For this review, take the finished solid that the model builds, in its own axes (mm). A direction names the side the tool comes from. Give positions to 0.01 mm unless a question says otherwise; leave off trailing zeros. Write each loop counter-clockwise with the first axis right and the second up, starting at its lowest first coordinate (ties: lowest second). Pieces come first, ordered by that corner, then holes. Notation, with made-up numbers: M 28,39.5 L 38,39.5 A21 ccw 38,58.5 Z; hole C -33.5,62.25 d2. An arc over 180 degrees is marked long. Answer as a JSON object with one key per item and string values. Group by question number.
```python
from build123d import *

# Parameters (mm, degrees)
SKETCH_1_W          = 95
SKETCH_1_H          = 45.5
EXTRUDE_1_DEPTH     = 2
SKETCH_2_W          = 7
SKETCH_2_H          = 2
CUT_EXTRUDE_1_DEPTH = 106.352978126
SKETCH_3_R          = 0.5
CUT_EXTRUDE_2_DEPTH = 106.352978126
SKETCH_5_W          = 13.5
SKETCH_5_H          = 24.5
CUT_EXTRUDE_3_DEPTH = 106.352978126
SKETCH_6_W          = 2
SKETCH_6_H          = 7
EXTRUDE_2_DEPTH     = 2
SKETCH_7_R          = 1.6
CUT_EXTRUDE_4_DEPTH = 2


with BuildPart() as part:
    # 草图1 → 凸台-拉伸1 (new body)
    with BuildSketch(Plane.XY):
        with Locations((47.5, 22.75)):
            Rectangle(SKETCH_1_W, SKETCH_1_H)
    extrude(amount=EXTRUDE_1_DEPTH)

    # 草图2 → 切除-拉伸1 (cut, through all)
    with BuildSketch(Plane.XY.offset(2)):
        with Locations((58.5, 44.5)):
            Rectangle(SKETCH_2_W, SKETCH_2_H)
        with Locations((36.5, 44.5)):
            Rectangle(SKETCH_2_W, SKETCH_2_H)
        with Locations((14.5, 44.5)):
            Rectangle(SKETCH_2_W, SKETCH_2_H)
        with Locations((80.5, 44.5)):
            Rectangle(SKETCH_2_W, SKETCH_2_H)
        with Locations((36.5, 1)):
            Rectangle(SKETCH_2_W, SKETCH_2_H)
        with Locations((58.5, 1)):
            Rectangle(SKETCH_2_W, SKETCH_2_H)
        with Locations((80.5, 1)):
            Rectangle(SKETCH_2_W, SKETCH_2_H)
    extrude(amount=-CUT_EXTRUDE_1_DEPTH, mode=Mode.SUBTRACT)

    # 草图3 → 切除-拉伸2 (cut, through all)
    with BuildSketch(Plane.XY.offset(2)):
        with Locations((11, 43.5)):
            Circle(SKETCH_3_R)
    cut_extrude_2 = extrude(amount=-CUT_EXTRUDE_2_DEPTH, mode=Mode.SUBTRACT)

    # 草图5 → 切除-拉伸3 (cut, through all)
    with BuildSketch(Plane.XY.offset(2)):
        with Locations((6.75, 12.25)):
            Rectangle(SKETCH_5_W, SKETCH_5_H)
    extrude(amount=-CUT_EXTRUDE_3_DEPTH, mode=Mode.SUBTRACT)

    # 草图6 → 凸台-拉伸2 (add)
    with BuildSketch(Plane.XY.offset(2)):
        with Locations((-1, 35)):
            Rectangle(SKETCH_6_W, SKETCH_6_H)
        with Locations((96, 32)):
            Rectangle(SKETCH_6_W, SKETCH_6_H)
        with Locations((96, 13.5)):
            Rectangle(SKETCH_6_W, SKETCH_6_H)
    extrude(amount=-EXTRUDE_2_DEPTH)

    # 草图阵列1: 切除-拉伸2 at 19 more places
    with Locations((7, 0, 0), (22, 0, 0), (29, 0, 0), (44, 0, 0), (51, 0, 0), (66, 0, 0), (73, 0, 0), (73, -41.5, 0), (66, -41.5, 0), (51, -41.5, 0), (44, -41.5, 0), (29, -41.5, 0), (22, -41.5, 0), (-11, -12, 0), (84, -8, 0), (-11, -5, 0), (84, -15, 0), (84, -26.5, 0), (84, -33.5, 0)):
        add(cut_extrude_2, mode=Mode.SUBTRACT)

    # 草图7 → 切除-拉伸4 (cut)
    with BuildSketch(Plane.XY.offset(2)):
        with Locations((6.75, 40.5)):
            Circle(SKETCH_7_R)
        with Locations((22.75, 13)):
            Circle(SKETCH_7_R)
    extrude(amount=-CUT_EXTRUDE_4_DEPTH, mode=Mode.SUBTRACT)


solid = part.part
```
Item 1: Consider section A-A (x = 6.75). Give the boundary of the cut face in (y, z), plus the area to 3 significant figures.
Item 2: Insertion check: P1, Ø1.2, axis at y = 1, z = 1.5, coming from the -X side; P2, Ø0.8, axis at y = 44.5, z = 1, coming from the +X side; P3, Ø1, axis at y = 40.5, z = 0.5, coming from the -X side. Each pin has a flat end and moves straight along its axis. Give the tip position at first contact, or say it passes through.
Item 3: Draft analysis for pull direction X (two halves, no side actions). For faces 1 (the flat face through (89, 0, 1)), 2 (the flat face through (36, 43.5, 1)), 3 (the flat face through (0, 42, 1)), state which applies: released by +X, released by -X, zero draft, split by the parting line, or undercut.
Item 4: Consider section B-B (z = 0.7). State how many separate pieces and enclosed holes the cut face has, plus the area to 3 significant figures.
Item 5: To check wall thickness, follow probe 1 along Y at (x, z) = (81, 1.75); probe 2 along X at (y, z) = (37.5, 1.75); probe 3 along X at (y, z) = (22, 1.5). State the ranges of each line that lie inside material, in increasing order.
Item 6: Machinability: for faces 4 (the flat face through (80, 2, 1)), 5 (the flat face through (95, 41, 1)), 6 (the flat face through (14, 43.5, 1)), which of the approach directions +Z, -Z, +X, -X, +Y, -Y give a long, thin tool a straight path to every point of the face, cutting with its end or side? Answer none if there is none.
Item 7: Consider section C-C (y = 27). Give the boundary of the cut face in (x, z).
Result set:
{
 "1": {"outline": "M 24.5,0 L 38.9,0 L 38.9,2 L 24.5,2 Z; M 42.1,0 L 45.5,0 L 45.5,2 L 42.1,2 Z", "area": "35.6 mm^2"},
 "2": {"P1": "stops at x = 13.5", "P2": "stops at x = 95", "P3": "stops at x = 0"},
 "3": {"face 1": "zero draft", "face 2": "undercut", "face 3": "released by -X"},
 "4": {"separate pieces": "1", "enclosed holes": "2", "area": "3,910 mm^2"},
 "5": {"probe 1": "y = 2 to 43.5", "probe 2": "x = -2 to 95", "probe 3": "x = 13.5 to 95"},
 "6": {"face 4": "+Z, -Z, -Y", "face 5": "+Z, -Z, +X, +Y", "face 6": "+Z, -Z, +Y"},
 "7": {"outline": "M 0,0 L 95,0 L 95,2 L 0,2 Z"}
}
